Source: CAD feature listing. Evaluate the final solid. Frame: model axes, mm. A direction names the side the tool comes from. Give positions to 0.01 mm unless a question says otherwise; leave off trailing zeros. Write each loop counter-clockwise with the first axis right and the second up, starting at its lowest first coordinate (ties: lowest second). Pieces come first, ordered by that corner, then holes. Notation, with made-up numbers: M 28,52 L 66,52 A37 cw 66,91 Z; hole C 58.5,21.5 d3. An arc over 180 degrees is marked long. Use CSV: the item, a comma, the result in double quotes. Start each with the question number.
from build123d import *

# Parameters (mm, degrees)
CROQUIS1_W              = 30
CROQUIS1_H              = 15
SALIENTE_EXTRUIR1_DEPTH = 2.5
CROQUIS2_W              = 25
CROQUIS2_H              = 15
SALIENTE_EXTRUIR2_DEPTH = 20
CORTAR_EXTRUIR1_DEPTH   = 20
CROQUIS5_R              = 5
CORTAR_EXTRUIR3_DEPTH   = 4.6


with BuildPart() as part:
    # Croquis1 → Saliente-Extruir1 (new body)
    with BuildSketch(Plane.XY):
        Rectangle(CROQUIS1_W, CROQUIS1_H)
    extrude(amount=SALIENTE_EXTRUIR1_DEPTH)

    # Croquis2 → Saliente-Extruir2 (add)
    with BuildSketch(Plane.XY.offset(2.5)):
        Rectangle(CROQUIS2_W, CROQUIS2_H)
    extrude(amount=SALIENTE_EXTRUIR2_DEPTH)

    # Croquis4 → Cortar-Extruir1 (cut)
    with BuildSketch(Plane(origin=(0, 7.5, 0), x_dir=(1, 0, 0), z_dir=(0, 1, 0))):
        Polygon((-12.5, -22.5), (0, -19.5), (12.5, -22.5), align=None)
    extrude(amount=-CORTAR_EXTRUIR1_DEPTH, mode=Mode.SUBTRACT)

    # Croquis5 → Cortar-Extruir3 (cut)
    with BuildSketch(Plane(origin=(0, 0, 0), x_dir=(-1, 0, 0), z_dir=(0, 0, -1))):
        with Locations((-7, 0)):
            Circle(CROQUIS5_R)
        with Locations((7, 0)):
            Circle(CROQUIS5_R)
    extrude(amount=-CORTAR_EXTRUIR3_DEPTH, mode=Mode.SUBTRACT)


solid = part.part
Item 1: Material intervals for probe 1 along Y at (x, z) = (-7, 3.5); probe 2 along X at (y, z) = (3, 2); probe 3 along X at (y, z) = (5.5, 12.75), sorted ascending.
Item 2: Pull-direction query (Y, two-part tool) for faces 1 (the flat face through (-7, 0, 4.6)), 2 (the flat face through (0, 7.5, 11)), 3 (the flat face through (6.16, 0.11, 20.98)); classes: released by +Y, released by -Y, zero draft, split by the parting line, or undercut.
Item 3: Set-up query: faces 4 (the flat face through (-6.34, 0.11, 21.02)), 5 (the flat face through (-12.5, 0, 12)), 6 (the flat face through (14, 0, 2.5)), 7 (the flat face through (7, 0, 4.6)). Return all of +Z, -Z, +X, -X, +Y, -Y with unobstructed straight access to the full face (end or side cutting, diameter ignored); none if empty.
Item 4: Section B-B (y = -3). Return the cut outline in (x, z).
Item 5: Section A-A (x = 7). Return the cut outline in (y, z), plus the area to 3 significant figures.
Item 6: Section C-C (x = -3). Return the cut outline in (y, z).
Item 7: Contact query for flat-ended pins moving along their axis: pin 1 Ø3 at (y, z) = (-1.5, 17) entering from -X; pin 2 Ø4 at (x, y) = (2, -4) entering from +Z; pin 3 Ø9 at (x, y) = (7, 0) entering from -Z; pin 4 Ø5 at (x, y) = (6.5, 5) entering from -Z. Output: stop coordinate, or through.
Item 8: Section D-D (z = 8.25). Return the cut outline in (x, y).
Output values:
1,probe 1,"y = -7.5 to -5, 5 to 7.5"
1,probe 2,"x = -15 to -11, -3 to 3, 11 to 15"
1,probe 3,"x = -12.5 to 12.5"
2,face 1,"undercut"
2,face 2,"released by +Y"
2,face 3,"zero draft"
3,face 4,"+Z, +Y, -Y"
3,face 5,"+Z, -X, +Y, -Y"
3,face 6,"+Z, +X, +Y, -Y"
3,face 7,"-Z"
4,outline,"M -15,0 L -11,0 L -11,4.6 L -3,4.6 L -3,0 L 3,0 L 3,4.6 L 11,4.6 L 11,0 L 15,0 L 15,2.5 L 12.5,2.5 L 12.5,22.5 L 0,19.5 L -12.5,22.5 L -12.5,2.5 L -15,2.5 Z"
5,outline,"M -7.5,0 L -5,0 L -5,4.6 L 5,4.6 L 5,0 L 7.5,0 L 7.5,21.18 L -7.5,21.18 Z"
5,area,"272 mm2"
6,outline,"M -7.5,0 L -3,0 L -3,4.6 L 3,4.6 L 3,0 L 7.5,0 L 7.5,20.22 L -7.5,20.22 Z"
7,pin 1,"stops at x = -12.5"
7,pin 2,"stops at z = 20.46"
7,pin 3,"stops at z = 4.6"
7,pin 4,"stops at z = 0"
8,outline,"M -12.5,-7.5 L 12.5,-7.5 L 12.5,7.5 L -12.5,7.5 Z"
